Geometry check sheet. Reference: the model listing, model coordinates, mm. A direction names the side the tool comes from. Give positions to 0.01 mm unless a question says otherwise; leave off trailing zeros. Order: outer loops, then holes, each group sorted by start corner. A loop starts at its lowest first (then second) coordinate and runs counter-clockwise, first axis right, second up.
Autodesk Inventor part; units mm, degrees
ref_plane "YZ Plane" through (0, 0, 0) normal (1, 0, 0) x (0, 1, 0)
ref_plane "XZ Plane" through (0, 0, 0) normal (0, 1, 0) x (-1, 0, 0)
ref_plane "XY Plane" through (0, 0, 0) normal (0, 0, 1) x (1, 0, 0)
sketch "Эскиз1" plane through (0, 0, 0) normal (0, 1, 0) x (-1, 0, 0)
  line L0 (-48.5, 38.5) -> (48.5, 38.5)
  line L1 (48.5, 38.5) -> (48.5, -38.5)
  line L2 (48.5, -38.5) -> (-48.5, -38.5)
  line L3 (-48.5, -38.5) -> (-48.5, 38.5)
  line L4 (-48.5, 38.5) -> (48.5, -38.5) construction
  line L5 (48.5, 38.5) -> (-48.5, -38.5) construction
  point P0 (0, 0)
  dimension "d0" = 77
  dimension "d1" = 97
extrude "Выдавливание1" add sketch "Эскиз1" along normal blind 1
sketch "Эскиз2" plane through (0, 1, 0) normal (0, 1, 0) x (1, 0, 0)
  line L0 (48.5, 38.5) -> (-48.5, 38.5)
  line L1 (-47, 38.5) -> (47, 38.5)
  line L2 (47, 38.5) -> (47, -35.5)
  line L3 (47, -35.5) -> (-47, -35.5)
  line L4 (-47, -35.5) -> (-47, 38.5)
  line L5 (0, 38.5) -> (0, 0)
  line L6 (-48.5, -38.5) -> (48.5, -38.5)
  dimension "d4" = 94
  dimension "d5" = 3
extrude "Выдавливание2" add sketch "Эскиз2" along normal blind 2
sketch "Эскиз3" plane through (0, 3, 0) normal (0, 1, 0) x (1, 0, 0)
  line L0 (47, 38.5) -> (-47, 38.5)
  line L1 (47, 38.5) -> (47, -35.5)
  line L2 (-47, 38.5) -> (47, 38.5)
  line L3 (47, 38.5) -> (47, 35.5)
  line L4 (47, 35.5) -> (-47, 35.5)
  line L5 (-47, 35.5) -> (-47, 38.5)
  point P0 (0, 0)
  dimension "d8" = 3
extrude "Выдавливание3" add sketch "Эскиз3" along normal blind 25
properties part number "Крышка Корпуса3"
Item 1: Sectioned sample at A-A (x = -10). Enter the section's corners in (y, z), and give its area (3 significant figures).
Reported:
outline: (0, -38.5) - (28, -38.5) - (28, -35.5) - (3, -35.5) - (3, 35.5) - (1, 35.5) - (1, 38.5) - (0, 38.5) - close
area: 300 mm2
Item 2: Draft check along X on faces 3 (the flat face through (-47, 2, -12)), 4 (the flat face through (47, 2, -13)), 5 (the flat face through (1, 14, -38.5)). Enter one of: released by +X, released by -X, zero draft, split by the parting line, or undercut.
Reported:
face 3: released by -X
face 4: released by +X
face 5: zero draft
Item 3: Sectioned sample at C-C (y = 8). Enter the section's corners in (x, z).
Reported:
outline: (-47, -38.5) - (47, -38.5) - (47, -35.5) - (-47, -35.5) - close
Item 4: Scan lines: L1, parallel to Y at x = 7, z = 18.5; L2, parallel to Z at x = -30, y = 14.25; L3, parallel to Z at x = -40, y = 2.75. Record each from-to range of solid material in increasing order.
Reported:
L1: y = 0 to 3
L2: z = -38.5 to -35.5
L3: z = -38.5 to 35.5
Item 5: Gauge pin test, flat ends, axial feed: pin 1 (10 mm diameter, centred on x = -2.5, y = 20, fed in from +Z); pin 2 (1 mm diameter, centred on x = 27.5, z = 12, fed in from +Y); pin 3 (0.6 mm diameter, centred on x = -5.5, y = 2, fed in from +Z); pin 4 (8 mm diameter, centred on y = 9, z = -8.5, fed in from -X). Record the tip position at first contact, or that the pin passes through.
Reported:
pin 1: stops at z = -35.5
pin 2: stops at y = 3
pin 3: stops at z = 35.5
pin 4: passes through
Item 6: Sectioned sample at B-B (z = 22.5). Enter the section's corners in (x, y), and give its area (3 significant figures).
Reported:
outline: (-48.5, 0) - (48.5, 0) - (48.5, 1) - (47, 1) - (47, 3) - (-47, 3) - (-47, 1) - (-48.5, 1) - close
area: 285 mm2
Item 7: Set-up check for faces 1 (the flat face through (1, 2, 35.5)), 2 (the flat face through (1, 0, 1)): record each of +Z, -Z, +X, -X, +Y, -Y from which the full face is reachable in a straight line by a thin tool's end or side.
Reported:
face 1: +Z, +X, -X, +Y
face 2: +Z, -Z, +X, -X, -Y
